Build history of the part. All positions in model axes, mm. A direction names the side the tool comes from. Coordinates: 2 decimals unless noted, no trailing zeros. Order: outer loops, then holes, each group sorted by start corner. A loop starts at its lowest first (then second) coordinate and runs counter-clockwise, first axis right, second up. Notation, with made-up numbers: (30.5, -23.75) -> (82.5, -23.75) arc R19 cw to (82.5, 9.25) -> close; hole circle Ø4 at (-4.5, 78.25). An arc over 180 degrees is marked (long way). Write each question's results on one line, items separated by ' | '.
from build123d import *

# Parameters (mm, degrees)
SKETCH1_R           = 0.5
BOSS_EXTRUDE1_DEPTH = 3
FILLET1_R           = 3
SKETCH2_R           = 2.5
CUT_EXTRUDE1_DEPTH  = 3


with BuildPart() as part:
    # Sketch1 → Boss-Extrude1 (new body)
    with BuildSketch(Plane.XY):
        Polygon((-10, 10), (0, 10), (10, 6.5), (10, 1.5), (6, 1.5), (6, -1.5), (10, -1.5), (10, -6.5), (0, -10), (-10, -10), align=None)
        with Locations((-5, 6.5)):
            Circle(SKETCH1_R, mode=Mode.SUBTRACT)
        with Locations((-5, -6.5)):
            Circle(SKETCH1_R, mode=Mode.SUBTRACT)
    extrude(amount=BOSS_EXTRUDE1_DEPTH)

    # Fillet1
    fillet1_edges = [part.edges().sort_by_distance(p)[0] for p in [
        (-10, 10, 1.5),
        (-10, -10, 1.5),
    ]]
    fillet(fillet1_edges, radius=FILLET1_R)

    # Sketch2 → Cut-Extrude1 (cut)
    with BuildSketch(Plane.XY.offset(3)):
        with Locations((-5, 0)):
            Circle(SKETCH2_R)
    extrude(amount=-CUT_EXTRUDE1_DEPTH, mode=Mode.SUBTRACT)


solid = part.part
Item 1: Slice it at A-A, the plane y = -2. List the corners of the cut face in (x, z).
Answer:
outline: (-10, 0) -> (-6.5, 0) -> (-6.5, 3) -> (-10, 3) -> close; (-3.5, 0) -> (10, 0) -> (10, 3) -> (-3.5, 3) -> close
Item 2: Pull direction X, two halves, no side cores. Call faces 1 (the cylindrical face through (-5, -7, 1)), 2 (the cylindrical face through (-2.615, 0.751, 1.521)), 3 (the cylindrical face through (-9.14, -9.1, 1.52)), 4 (the flat face through (10, 4, 1)): released by +X, released by -X, zero draft, split by the parting line, or undercut.
Answer:
face 1: undercut | face 2: undercut | face 3: released by -X | face 4: released by +X
Item 3: Pin check, flat tips, straight feed: pin 1 (0.9 mm diameter, centred on x = 9, z = 1.5, fed in from +Y); pin 2 (1.5 mm diameter, centred on x = 2, z = 0.5, fed in from +Y). Stop position of each tip, or through.
Answer:
pin 1: stops at y = 7.01 | pin 2: stops at y = 9.56
Item 4: Slice it at D-D, the plane y = 0. List the corners of the cut face in (x, z), and give its area (3 significant figures).
Answer:
outline: (-10, 0) -> (-7.5, 0) -> (-7.5, 3) -> (-10, 3) -> close; (-2.5, 0) -> (6, 0) -> (6, 3) -> (-2.5, 3) -> close | area: 33.0 mm^2
Item 5: Slice it at B-B, the plane x = -5. List the corners of the cut face in (y, z), and give its area (3 significant figures).
Answer:
outline: (-10, 0) -> (-7, 0) -> (-7, 3) -> (-10, 3) -> close; (-6, 0) -> (-2.5, 0) -> (-2.5, 3) -> (-6, 3) -> close; (2.5, 0) -> (6, 0) -> (6, 3) -> (2.5, 3) -> close; (7, 0) -> (10, 0) -> (10, 3) -> (7, 3) -> close | area: 39.0 mm^2
Item 6: Tool access for faces 5 (the flat face through (6, 0, 1)), 6 (the flat face through (-10, 0, 1)): list every direction of +Z, -Z, +X, -X, +Y, -Y with a clear straight run to the whole face (end or side of a thin tool).
Answer:
face 5: +Z, -Z, +X | face 6: +Z, -Z, -X, +Y, -Y
Item 7: Drill centre lines: line 1 (Y direction, x = -5, z = 1.5); line 2 (X direction, y = -6.25, z = 1.35); line 3 (Y direction, x = 7, z = 2.85). Where is each one in solid material? Low to high. Write a range as from..to.
Answer:
line 1: y = -10..-7, -6..-2.5, 2.5..6, 7..10 | line 2: x = -10..-5.43, -4.57..10 | line 3: y = -7.55..-1.5, 1.5..7.55
Item 8: Slice it at C-C, the plane z = 1.85. List the corners of the cut face in (x, y), and give its area (3 significant figures).
Answer:
outline: (-10, -7) arc R3 ccw to (-7, -10) -> (0, -10) -> (10, -6.5) -> (10, -1.5) -> (6, -1.5) -> (6, 1.5) -> (10, 1.5) -> (10, 6.5) -> (0, 10) -> (-7, 10) arc R3 ccw to (-10, 7) -> close; hole circle Ø5 at (-5, 0); hole circle Ø1 at (-5, -6.5); hole circle Ø1 at (-5, 6.5) | area: 328 mm^2
